```python
from build123d import *

# Parameters (mm, degrees)
SKETCH_264_W = 30
SKETCH_264_H = 55


with BuildPart() as part:
    # По траектории2: sweep along a path in Sketch 339
    with BuildLine(Plane(origin=(0, 0, 0), x_dir=(0, 0, -1), z_dir=(1, 0, 0))) as sweep_2_path:
        Line((0, 0), (37, 0))
        ThreePointArc((37, 0), (67, 8.038475773), (88.961524227, 30))
        ThreePointArc((88.961524227, 30), (168.942963927, 53.05548357), (194.997071793, -26))
        ThreePointArc((194.997071793, -26), (201.894019343, -89.07186966), (261.54579658, -110.688856044))
    # Sketch 264 → По траектории2 (sweep)
    with BuildSketch(Plane.XY):
        Rectangle(SKETCH_264_W, SKETCH_264_H)
    sweep(path=sweep_2_path.line)


solid = part.part
```
Geometry: final body of the model. Coordinates: model frame, mm. A direction names the side the tool comes from. Coordinates: 2 decimals unless noted, no trailing zeros. Loops run counter-clockwise (first coordinate to the right, second up) from the corner with the lowest first, then second, coordinate; pieces in that order, holes last. Notation, with made-up numbers: (41.5, 21) -> (79.5, 21) arc R5 cw to (79.5, 27) -> close; hole circle Ø3 at (2.5, 20.25). An arc over 180 degrees is marked (long way). Use a Markdown table: item, result. Add a question column.
(1) Section query A-A, the plane y = 0. Return loops of the section in (x, z), plus the area to 3 significant figures.
(2) Mould query, pull axis Z, two halves, no side actions, for faces 1 (the flat face through (-0.21, -111.065, -261.626)), 2 (the flat face through (-15, 26, -165)), 3 (the cylindrical face through (-0.21, -71.68, -223.207)), 4 (the cylindrical face through (-0.21, 78.23, -180.12)). Classes: pulls with the +Z half, pulls with the -Z half, needs draft (parallel to the pull), parting line crosses it, or undercut.
(3) Section query B-B, the plane x = -10. Return loops of the section in (y, z), plus the area to 3 significant figures.
(4) Section query C-C, the plane z = -208. Return loops of the section in (x, y).
(5) Pin query (flat end, axial travel): pin 1 Ø10 at (x, y) = (-0.5, 36.5) entering from +Z; pin 2 Ø12 at (x, y) = (2.5, 54) entering from +Z; pin 3 Ø15 at (x, z) = (6, -14.5) entering from -Y. Return the tip coordinate at first contact, or that it passes through.
(6) Access query for faces 5 (the flat face through (0, 27.5, -19)), 6 (the flat face through (0, -27.5, -19)), 7 (the cylindrical face through (0.21, -16.1, -80.19)). Directions: +Z, -Z, +X, -X, +Y, -Y. A direction counts if a zero-diameter tool reaches every point of the face in a straight line with its end or side. Return the directions, or none.
(7) Section query D-D, the plane y = -41.5. Return loops of the section in (x, z).
(8) Line query: line 1 along Y through (x, z) = (6, -24.5); line 2 along Z through (x, y) = (-1.75, -9); line 3 along Z through (x, y) = (-10.25, 8). Output: solid intervals per line, ascending.
Answer:
| question | item | result |
|---|---|---|
| 1 | outline | (-15, -228.42) -> (15, -228.42) -> (15, -173.42) -> (-15, -173.42) -> close; (-15, -100.69) -> (15, -100.69) -> (15, 0) -> (-15, 0) -> close |
| 1 | area | 4,670 mm^2 |
| 2 | face 1 | pulls with the -Z half |
| 2 | face 2 | needs draft |
| 2 | face 3 | undercut |
| 2 | face 4 | parting line crosses it |
| 3 | outline | (-137.59, -267.26) -> (-83.79, -255.83) arc R32.5 cw to (-37.92, -219.78) arc R87.5 ccw to (43.75, -65.15) arc R32.5 cw to (27.5, -37) -> (27.5, 0) -> (-27.5, 0) -> (-27.5, -37) arc R87.5 ccw to (16.25, -112.78) arc R32.5 cw to (-14.08, -170.21) arc R87.5 ccw to start |
| 3 | area | 23,000 mm^2 |
| 4 | outline | (-15, -129.26) -> (15, -129.26) -> (15, 56.19) -> (-15, 56.19) -> close |
| 5 | pin 1 | stops at z = -52.62 |
| 5 | pin 2 | stops at z = -67.76 |
| 5 | pin 3 | stops at y = -27.5 |
| 6 | face 5 | +Z, +X, -X, +Y |
| 6 | face 6 | +Z, +X, -X, -Y |
| 6 | face 7 | +X, -X, -Y |
| 7 | outline | (-15, -218.31) -> (15, -218.31) -> (15, -162.2) -> (-15, -162.2) -> close |
| 8 | line 1 | y = -27.5 to 27.5 |
| 8 | line 2 | z = -227.96 to -172.15, -90.81 to 0 |
| 8 | line 3 | z = -228.06 to -172.42, -107.37 to 0 |
